Model file for the job. Use its own axes, mm. A direction names the side the tool comes from. Round coordinates to 2 decimals unless told otherwise and drop trailing zeros. Loops run counter-clockwise (first coordinate to the right, second up) from the corner with the lowest first, then second, coordinate; pieces in that order, holes last. Notation, with made-up numbers: (-29, 30.25) -> (-20, 30.25) arc R24 ccw to (-20, 63.25) -> close; hole circle Ø1 at (-23, 49.25). An arc over 180 degrees is marked (long way). Use a Markdown table: item, result.
from build123d import *

# Parameters (mm, degrees)
EXTRUDE_1_DEPTH        = 21
EXTRUDE_2_DEPTH        = 3
FILLET_1_R             = 4
FILLET_1_OF_MIRROR_2_R = 4
CUT_EXTRUDE_1_DEPTH    = 5
EXTRUDE_3_DEPTH        = 4.75


with BuildPart() as part:
    # Эскиз1 → Бобышка-Вытянуть1 (new body, symmetric)
    with BuildSketch(Plane.XY):
        Polygon((0, 42), (0, 0), (42, 0), (42, 4), (4, 4), (4, 42), align=None)
    extrude(amount=EXTRUDE_1_DEPTH, both=True)

    # Эскиз2 → Бобышка-Вытянуть2 (add)
    with BuildSketch(Plane.XY.offset(21)):
        Polygon((42, 4), (4, 4), (4, 42), (8, 42), (42, 8), align=None)
    extrude_2 = extrude(amount=-EXTRUDE_2_DEPTH)

    # Скругление1
    fillet_1_edges = [part.edges().sort_by_distance(p)[0] for p in [
        (8, 42, 19.5),
        (42, 8, 19.5),
    ]]
    fillet(fillet_1_edges, radius=FILLET_1_R)

    # Зеркальное отражение2: Бобышка-Вытянуть2 across plane
    add(extrude_2.mirror(Plane.XY))

    # Скругление1 of Зеркальное отражение2
    fillet_1_of_mirror_2_edges = [part.edges().sort_by_distance(p)[0] for p in [
        (8, 42, -19.5),
        (42, 8, -19.5),
    ]]
    fillet(fillet_1_of_mirror_2_edges, radius=FILLET_1_OF_MIRROR_2_R)

    # Эскиз3 → Вырез-Вытянуть1 (cut, through all)
    with BuildSketch(Plane(origin=(0, 4, 0), x_dir=(1, 0, 0), z_dir=(0, 1, 0))):
        with BuildLine():
            Line((20, 4), (23.611111111, 4))
            Line((23.611111111, 4), (26.030927835, 6.680412371))
            ThreePointArc((26.030927835, 6.680412371), (30.435916317, 7.733382425), (33, 4))
            Line((33, 4), (33, -4))
            ThreePointArc((33, -4), (30.435916317, -7.733382425), (26.030927835, -6.680412371))
            Line((26.030927835, -6.680412371), (23.611111111, -4))
            Line((23.611111111, -4), (20, -4))
            ThreePointArc((20, -4), (16, 0), (20, 4))
        make_face()
    cut_extrude_1 = extrude(amount=-CUT_EXTRUDE_1_DEPTH, mode=Mode.SUBTRACT)

    # Эскиз4 → Бобышка-Вытянуть3 (add, symmetric)
    with BuildSketch(Plane.XY):
        Polygon((1.232233047, 0), (0, -1.232233047), (1.767766953, -3), (4.767766953, 0), align=None)
        Polygon((42, 0), (39, -3), (37.232233047, -1.232233047), (38.464466094, 0), align=None)
    extrude_3 = extrude(amount=EXTRUDE_3_DEPTH, both=True)

    # Зеркальное отражение3: Вырез-Вытянуть1, Бобышка-Вытянуть3 across plane
    add(cut_extrude_1.mirror(Plane(origin=(0, 0, 0), x_dir=(0, 0, 1), z_dir=(-0.707106781, 0.707106781, 0))), mode=Mode.SUBTRACT)
    add(extrude_3.mirror(Plane(origin=(0, 0, 0), x_dir=(0, 0, 1), z_dir=(-0.707106781, 0.707106781, 0))))


solid = part.part
Q1. Band-saw the part on B-B, the plane y = 17.5. Give the cut face in (x, z).
Results list:
| item | result |
|---|---|
| outline | (0, -21) -> (32.5, -21) -> (32.5, -18) -> (4, -18) -> (4, -3.12) -> (0, -3.12) -> close; (0, 3.12) -> (4, 3.12) -> (4, 18) -> (32.5, 18) -> (32.5, 21) -> (0, 21) -> close |
Q2. Band-saw the part on D-D, the plane x = 2.5. Give the cut face in (y, z).
Results list:
| item | result |
|---|---|
| outline | (-2.27, -4.75) -> (0, -4.75) -> (0, -21) -> (42, -21) -> (42, 21) -> (0, 21) -> (0, 4.75) -> (-2.27, 4.75) -> close; hole (20, -4) -> (23.61, -4) -> (26.03, -6.68) arc R4 ccw to (33, -4) -> (33, 4) arc R4 ccw to (26.03, 6.68) -> (23.61, 4) -> (20, 4) arc R4 ccw to start |
Q3. Band-saw the part on C-C, the plane x = 19. Give the cut face in (y, z), plus the area to 3 significant figures.
Results list:
| item | result |
|---|---|
| outline | (0, -21) -> (31, -21) -> (31, -18) -> (4, -18) -> (4, -3.87) -> (0, -3.87) -> close; (0, 3.87) -> (4, 3.87) -> (4, 18) -> (31, 18) -> (31, 21) -> (0, 21) -> close |
| area | 299 mm² |
Q4. Tool access for faces 1 (the face through (22, 2, -4)), 2 (the face through (4, 22.7, 4.3)), 3 (the face through (-1.52, 3.25, -0.07)), 4 (the face through (2, -1, -4.75)), 5 (the face through (2.03, 30.5, 7.71)): list every direction of +Z, -Z, +X, -X, +Y, -Y with a clear straight run to the whole face (end or side of a thin tool).
Results list:
| item | result |
|---|---|
| face 1 | +Y, -Y |
| face 2 | +X, +Y |
| face 3 | +Z, -Z, -X |
| face 4 | -Z, +X, -X, -Y |
| face 5 | +X, -X |
Q5. Drill centre lines: L1, parallel to Z at x = 25, y = 11.5; L2, parallel to X at y = 15, z = -12.5. Where is each one in solid material? Low to high. Write a range as from..to.
Results list:
| item | result |
|---|---|
| L1 | z = -21..-18, 18..21 |
| L2 | x = 0..4 |
Q6. Band-saw the part on A-A, the plane z = 0. Give the cut face in (x, y), plus the area to 3 significant figures.
Results list:
| item | result |
|---|---|
| outline | (-3, 1.77) -> (-1.23, 0) -> (0, 1.23) -> (0, 0) -> (1.23, 0) -> (0, -1.23) -> (1.77, -3) -> (4.77, 0) -> (16, 0) -> (16, 4) -> (4, 4) -> (4, 16) -> (0, 16) -> (0, 4.77) -> close; (-3, 39) -> (-1.23, 37.23) -> (0, 38.46) -> (0, 33) -> (4, 33) -> (4, 42) -> (0, 42) -> close; (33, 0) -> (38.46, 0) -> (37.23, -1.23) -> (39, -3) -> (42, 0) -> (42, 4) -> (33, 4) -> close |
| area | 214 mm² |
Q7. Flat gauge pins, fed straight in: pin 1 (10 mm diameter, centred on y = 20.5, z = 11.5, fed in from -X); pin 2 (4 mm diameter, centred on x = 22.5, z = 14, fed in from +Y); pin 3 (0.9 mm diameter, centred on x = 39.5, y = -1, fed in from +Z); pin 4 (2.5 mm diameter, centred on x = -1, y = 40.5, fed in from -Z). Where does each tip first touch, or does it go through?
Results list:
| item | result |
|---|---|
| pin 1 | stops at x = 0 |
| pin 2 | stops at y = 4 |
| pin 3 | stops at z = 4.75 |
| pin 4 | stops at z = -21 |
Q8. Pull direction Y, two halves, no side cores. Call faces 6 (the face through (-1, 2, -4.75)), 7 (the face through (2, 22, -4)), 8 (the face through (0.87, -2.1, -0.07)), 9 (the face through (37.84, -0.625, 0.067)): released by +Y, released by -Y, zero draft, split by the parting line, or undercut.
Results list:
| item | result |
|---|---|
| face 6 | zero draft |
| face 7 | undercut |
| face 8 | released by -Y |
| face 9 | undercut |
